Verification items for this drawing (mm, ordinates from the low corner). A direction names the side the tool comes from. Coordinates: 2 decimals unless noted, no trailing zeros. Order: outer loops, then holes, each group sorted by start corner. A loop starts at its lowest first (then second) coordinate and runs counter-clockwise, first axis right, second up.
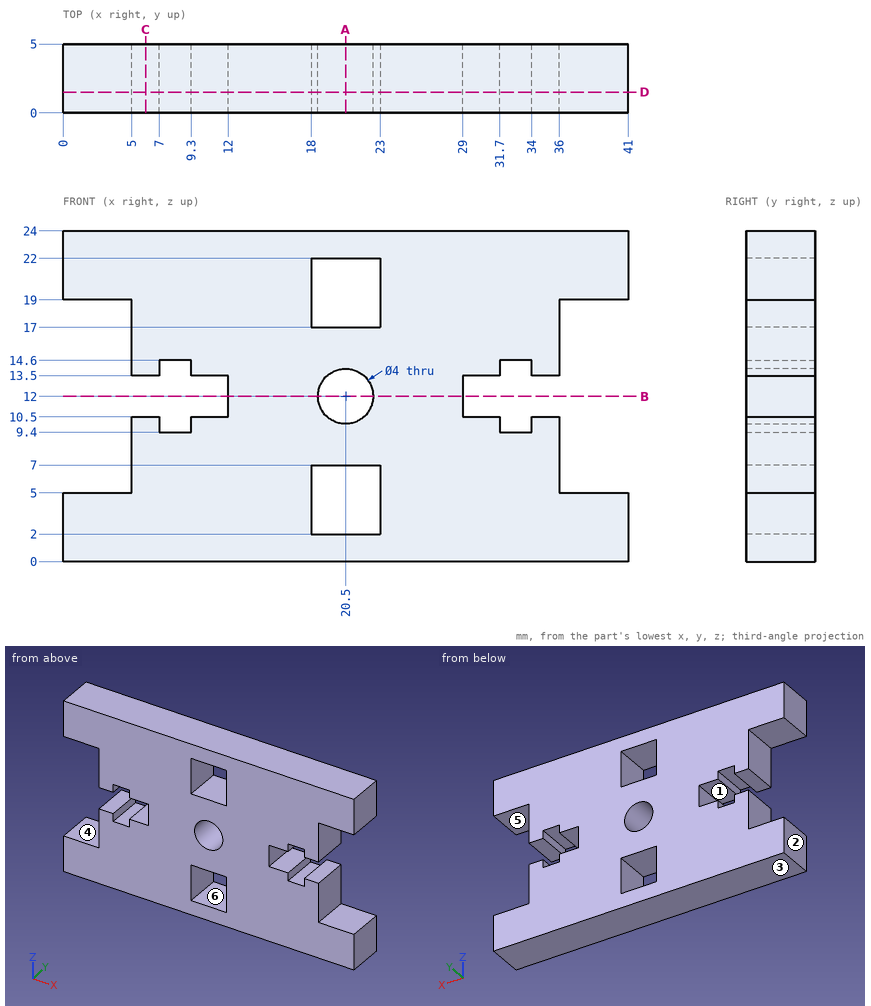
Item 1: Sectioned sample at A-A (x = 20.5). Record the cut outline in (y, z), and give its area (3 significant figures).
Item 2: Thickness scan on line 1 along Z through (x, y) = (38, 0.95); line 2 along X through (y, z) = (3.9, 12); line 3 along Z through (x, y) = (20, 1.95). Record the ranges inside material, lowest first.
Item 3: Release check for a two-part mould opening along Z. For the marked faces 1, 2 and 3 record: pulls with the +Z half, pulls with the -Z half, needs draft (parallel to the pull), parting line crosses it, or undercut.
Item 4: Depth check by flat-ended pin: P1, Ø0.9, axis at y = 1.5, z = 10, coming from the -X side; P2, Ø0.9, axis at y = 2, z = 14, coming from the +X side; P3, Ø0.9, axis at y = 3.5, z = 12.5, coming from the +X side. Enter the tip coordinate at first touch or a pass-through.
Item 5: Sectioned sample at B-B (z = 12). Record the cut outline in (x, y), and give its area (3 significant figures).
Item 6: Sectioned sample at D-D (y = 1.5). Give the number of separate pieces and of enclosed holes in the cut face, and give its area (3 significant figures).
Item 7: Tool access check on the marked faces 4, 5 and 6. Record the directions out of +Z, -Z, +X, -X, +Y, -Y that give a thin tool (end or side, any length) a straight path to the whole face; none if there is none.
Item 8: Sectioned sample at C-C (x = 6). Record the cut outline in (y, z).
Geometry check:
1. outline: (0, 0) - (5, 0) - (5, 2) - (0, 2) - close; (0, 7) - (5, 7) - (5, 10) - (0, 10) - close; (0, 14) - (5, 14) - (5, 17) - (0, 17) - close; (0, 22) - (5, 22) - (5, 24) - (0, 24) - close
1. area: 50.0 mm2
2. line 1: z = 0 to 5, 19 to 24
2. line 2: x = 12 to 18.5, 22.5 to 29
2. line 3: z = 0 to 2, 7 to 10.06, 13.94 to 17, 22 to 24
3. face 1: undercut
3. face 2: needs draft
3. face 3: pulls with the -Z half
4. P1: stops at x = 5
4. P2: stops at x = 36
4. P3: stops at x = 29
5. outline: (12, 0) - (18.5, 0) - (18.5, 5) - (12, 5) - close; (22.5, 0) - (29, 0) - (29, 5) - (22.5, 5) - close
5. area: 65.0 mm2
6. separate pieces: 1
6. enclosed holes: 3
6. area: 729 mm2
7. face 4: -X, +Y, -Y
7. face 5: +X, +Y, -Y
7. face 6: +Y, -Y
8. outline: (0, 0) - (5, 0) - (5, 10.5) - (0, 10.5) - close; (0, 13.5) - (5, 13.5) - (5, 24) - (0, 24) - close
